Work out the finished part from the listing and answer in its coordinate system (mm). Face numbers are marked on the shaded views. A direction names the side the tool comes from. Round coordinates to 2 decimals unless told otherwise and drop trailing zeros. Write each loop counter-clockwise with the first axis right and the second up, starting at its lowest first coordinate (ties: lowest second). Pieces come first, ordered by that corner, then holes.
1. A tool of negligible diameter and unlimited length cuts with its end or side. For the marked faces 1 and 2, from which of +Z, -Z, +X, -X, +Y, -Y can it reach the whole face along a straight path? Write none if from no direction.
2. Find section C-C (y = 34.2). Write down the section's boundary in (x, z).
3. Flat-ended cylindrical pins translate along their axes: pin 1 Ø15 at (y, z) = (18, -26.5) entering from +X; pin 2 Ø10 at (x, z) = (20, -63) entering from +Y; pin 3 Ø4 at (x, z) = (7.5, -43) entering from +Y. Find the tip coordinate at first contact, or state that the pin passes through.
4. Find section B-B (x = 2.4). Write down the section's boundary in (y, z), and give its area (3 significant figures).
5. Find section D-D (y = 19.5). Write down the section's boundary in (x, z).
6. Find section A-A (z = -67). Write down the section's boundary in (x, y), and give its area (3 significant figures).
7. Straight lines are drawn through the part: probe 1 along Z at (x, y) = (2.4, 19); probe 2 along Z at (x, y) = (2, 34); probe 3 along X at (y, z) = (8, -58). For each, find the intervals that lie inside material, in ascending order.
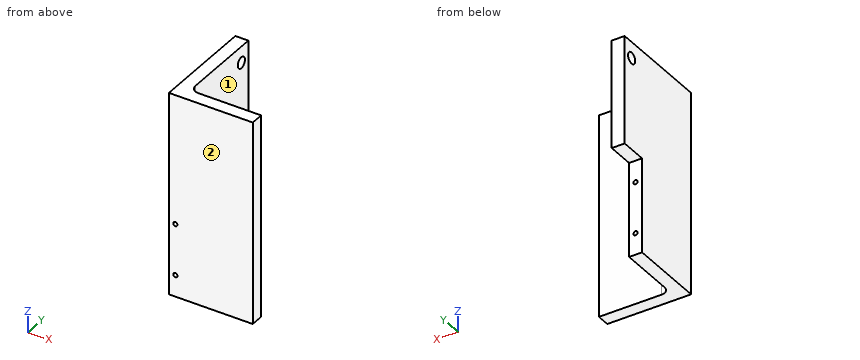
Autodesk Inventor part; units mm, degrees
ref_plane "YZ Plane" through (0, 0, 0) normal (1, 0, 0) x (0, 1, 0)
ref_plane "XZ Plane" through (0, 0, 0) normal (0, 1, 0) x (-1, 0, 0)
ref_plane "XY Plane" through (0, 0, 0) normal (0, 0, 1) x (1, 0, 0)
sketch "Sketch1" plane through (0, 0, 0) normal (0, 0, 1) x (1, 0, 0)
  line L0 (0, 38.2) -> (0, 0)
  line L1 (0, 0) -> (31, 0)
  line L2 (31, 0) -> (31, 4.8)
  line L3 (31, 4.8) -> (7.8, 4.8)
  line L4 (4.8, 7.8) -> (4.8, 38.2)
  line L5 (4.8, 38.2) -> (0, 38.2)
  arc A0 (4.8, 7.8) -> (7.8, 4.8) centre (7.8, 7.8) ccw
  dimension "d0" = 31
  dimension "d1" = 38.2
  dimension "d2" = 4.8
  dimension "d3" = 4.8
  dimension "d4" = 3
extrude "Extrusion1" add sketch "Sketch1" against normal blind 75
sketch "Sketch2" plane through (0, 0, 0) normal (-1, 0, 0) x (0, 0, 1)
  line L0 (0, 0) -> (0, 38.2)
  line L1 (0, 38.2) -> (-75, 38.2)
  point P0 (-6, 34.2)
  dimension "d7" = 4
  dimension "d8" = 6
hole "Hole1" at (0, 34.2, -6) direction (1, 0, 0) diameter 4.134 end through all
sketch "Sketch3" plane through (0, 0, 0) normal (-1, 0, 0) x (0, 0, 1)
  line L0 (0, 0) -> (0, 38.2)
  line L1 (0, 38.2) -> (-75, 38.2)
  line L2 (-100.4339, 50.496) -> (-40, 50.496)
  line L3 (-40, 50.496) -> (-40, 28.2)
  line L4 (-40, 28.2) -> (-100.4339, 28.2)
  line L5 (-100.4339, 28.2) -> (-100.4339, 50.496)
  dimension "d16" = 40
  dimension "d17" = 10
extrude "Extrusion2" cut sketch "Sketch3" against normal through all
sketch "Sketch4" plane through (0, 28.2, -40) normal (0, 1, 0) x (1, 0, 0)
  line L0 (0, 35) -> (4.8, 35)
  line L1 (0, 0) -> (4.8, 0)
  point P0 (0, -40)
  point P1 (2.4, 27)
  point P2 (2.4, 8)
  dimension "d20" = 8
  dimension "d21" = 8
  dimension "d22" = 19
hole "Hole2" at (2.4, 28.2, -67) at (2.4, 28.2, -48) direction (0, -1, 0) diameter 1.567 end through all
properties part number "Left Angle"
Worked answers:
1. face 1: +Z, -Z, +X, +Y
1. face 2: +Z, -Z, +X, -X, -Y
2. outline: (0, -40) - (4.8, -40) - (4.8, -8.07) - (0, -8.07) - close; (0, -3.93) - (4.8, -3.93) - (4.8, 0) - (0, 0) - close
3. pin 1: stops at x = 4.8
3. pin 2: stops at y = 4.8
3. pin 3: stops at y = 5.87
4. outline: (0, -75) - (28.2, -75) - (28.2, -67.78) - (0, -67.78) - close; (0, -66.22) - (28.2, -66.22) - (28.2, -48.78) - (0, -48.78) - close; (0, -47.22) - (28.2, -47.22) - (28.2, -40) - (38.2, -40) - (38.2, 0) - (0, 0) - close; hole circle Ø4.13 at (34.2, -6)
4. area: 2,410 mm2
5. outline: (0, -75) - (4.8, -75) - (4.8, 0) - (0, 0) - close; hole circle Ø1.57 at (2.4, -67); hole circle Ø1.57 at (2.4, -48)
6. outline: (0, 0) - (1.62, 0) - (1.62, 28.2) - (0, 28.2) - close; (3.18, 0) - (31, 0) - (31, 4.8) - (7.8, 4.8) arc R3 cw to (4.8, 7.8) - (4.8, 28.2) - (3.18, 28.2) - close
6. area: 219 mm2
7. probe 1: z = -75 to -67.78, -66.22 to -48.78, -47.22 to 0
7. probe 2: z = -40 to -8.06, -3.94 to 0
7. probe 3: x = 0 to 4.8
